For this review, take the finished solid that the model builds, in its own axes (mm). Face numbers are marked on the shaded views. Round coordinates to 2 decimals unless told otherwise and drop trailing zeros. Put each result on its own line as item: value.
from build123d import *

# Parameters (mm, degrees)
SKETCH1_W               = 130
SKETCH1_H               = 10
SKETCH1_R               = 0.9
SKETCH1_R_2             = 3
BOSS_EXTRUDE1_DEPTH     = 10
CUT_EXTRUDE1_DEPTH      = 131.766968306
CUT_EXTRUDE1_DEPTH_BACK = 131.766968306
SKETCH2_W               = 30
SKETCH2_H               = 2
FILLET1_R               = 5


with BuildPart() as part:
    # Sketch1 → Boss-Extrude1 (new body)
    with BuildSketch(Plane(origin=(0, 0, 0), x_dir=(1, 0, 0), z_dir=(0, 1, 0))):
        with Locations((65, 5)):
            Rectangle(SKETCH1_W, SKETCH1_H)
        with Locations(Location((3, 5, 0), (0, 0, 270))):
            Circle(SKETCH1_R, mode=Mode.SUBTRACT)
        with Locations(Location((53, 5, 0), (0, 0, 270))):
            Circle(SKETCH1_R, mode=Mode.SUBTRACT)
        with Locations(Location((125, 5, 0), (0, 0, 270))):
            Circle(SKETCH1_R_2, mode=Mode.SUBTRACT)
    extrude(amount=BOSS_EXTRUDE1_DEPTH)

    # Sketch2 → Cut-Extrude1 (cut, two sides: drawn at the far end of the back side and taken through both)
    with BuildSketch(Plane.XY.offset(-CUT_EXTRUDE1_DEPTH_BACK)):
        with Locations((28, 1)):
            Rectangle(SKETCH2_W, SKETCH2_H)
    extrude(amount=CUT_EXTRUDE1_DEPTH + CUT_EXTRUDE1_DEPTH_BACK, mode=Mode.SUBTRACT)

    # Fillet1
    fillet1_edges = [part.edges().sort_by_distance(p)[0] for p in [
        (130, 5, 0),
        (130, 5, -10),
        (0, 5, 0),
        (0, 5, -10),
    ]]
    fillet(fillet1_edges, radius=FILLET1_R - 0.0001)  # a hair under: the kernel refuses the full size


solid = part.part
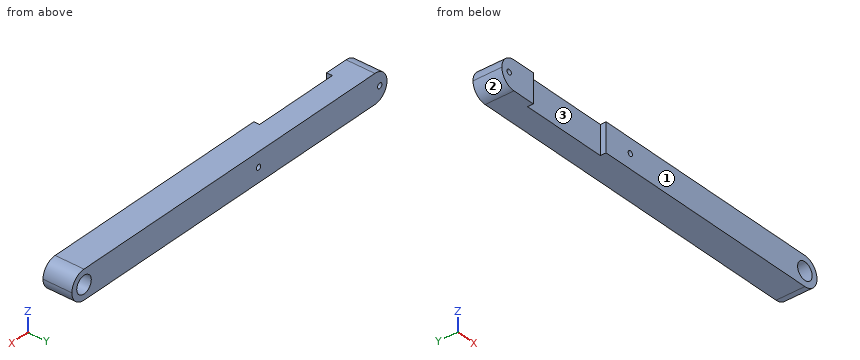
(1) Insertion check: pin 1 Ø0.6 at (y, z) = (1.5, -3) entering from -X; pin 2 Ø4 at (x, z) = (34, -1.5) entering from -Y; pin 3 Ø4 at (y, z) = (6, -7.5) entering from -X. Each pin has a flat end and moves straight along its axis. Give the tip position at first contact, or say it passes through.
A:
pin 1: stops at x = 0.3
pin 2: stops at y = 2
pin 3: stops at x = 0.03
(2) To check wall thickness, follow L1, parallel to X at y = 7.5, z = -5; L2, parallel to Z at x = 53, y = 7.25; L3, parallel to X at y = 0.5, z = -3.75. State the ranges of each line that lie inside material, in increasing order.
A:
L1: x = 0 to 2.1, 3.9 to 52.1, 53.9 to 122, 128 to 130
L2: z = -10 to -5.9, -4.1 to 0
L3: x = 0.16 to 13, 43 to 122.27, 127.73 to 129.84
(3) Draft analysis for pull direction X (two halves, no side actions). For the marked faces 1, 2 and 3, state which applies: released by +X, released by -X, zero draft, split by the parting line, or undercut.
A:
face 1: zero draft
face 2: released by -X
face 3: undercut
(4) Add section A-A on y = 7. State how many separate pieces and enclosed holes the cut face has, then the cut area to 3 significant figures.
A:
separate pieces: 1
enclosed holes: 3
area: 1,250 mm2
